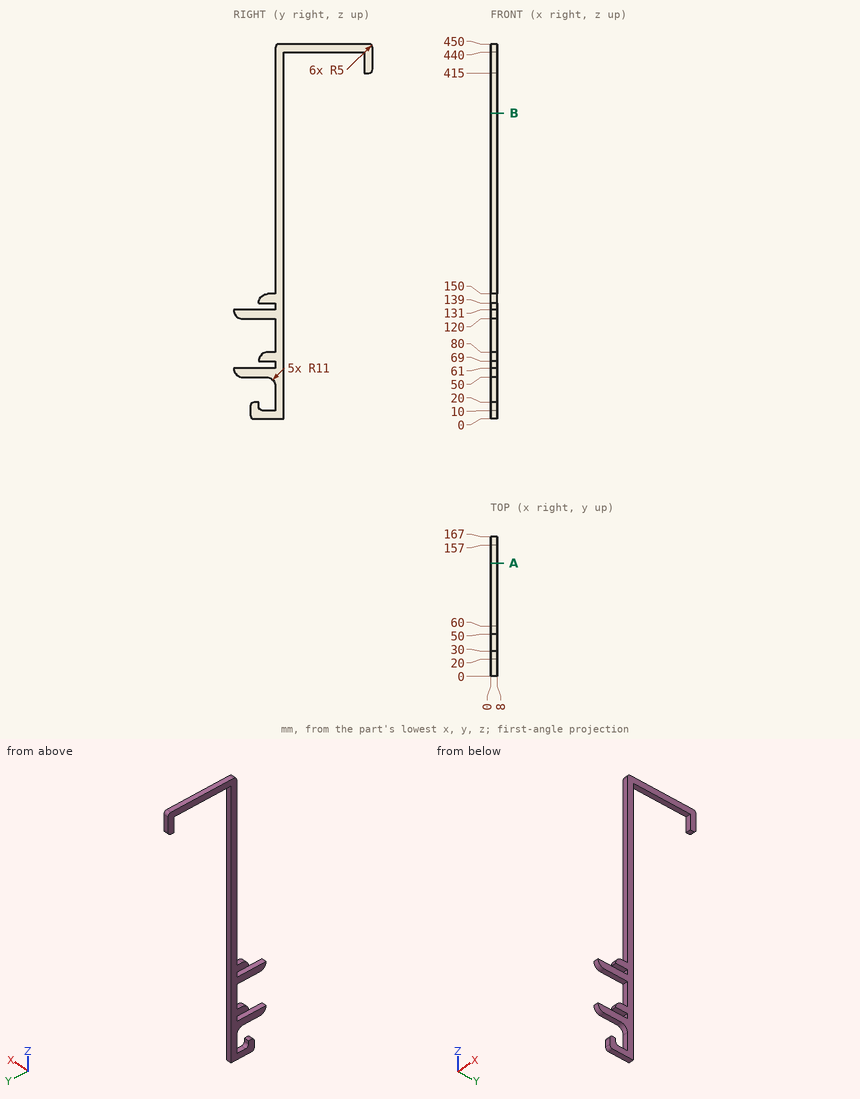
Design review of the part shown in the three views and the two pictorial views. Dimensions are in mm from the part's minimum x, y and z. Coordinates: 2 decimals unless noted, no trailing zeros. Loops run counter-clockwise (first coordinate to the right, second up) from the corner with the lowest first, then second, coordinate; pieces in that order, holes last.
Q1. We need section B-B on z = 367. State the section outline as (x, y) points, and give its area (3 significant figures).
Reported:
outline: (0, 50) - (8, 50) - (8, 60) - (0, 60) - close
area: 80.0 mm2
Q2. For pin 1 (3 mm diameter, centred on x = 5, y = 132.5, fed in from -Z); pin 2 (4 mm diameter, centred on x = 3.5, y = 160.5, fed in from -Z); pin 3 (2.5 mm diameter, centred on x = 4, z = 18, fed in from +Y), all flat-tipped, find the tip position at first contact; note any pin that passes through.
Reported:
pin 1: stops at z = 440
pin 2: stops at z = 415
pin 3: stops at y = 60
Q3. We need section A-A on y = 135.5. State the section outline as (x, z) points.
Reported:
outline: (0, 440) - (8, 440) - (8, 450) - (0, 450) - close
Q4. To check wall thickness, follow line 1 (Z direction, x = 6.25, y = 27); line 2 (Y direction, x = 0.5, z = 427); line 3 (Z direction, x = 6.75, y = 19.5). State the ranges of each line that lie inside material, in increasing order.
Reported:
line 1: z = 0 to 20, 50 to 61, 120 to 131
line 2: y = 50 to 60, 157 to 167
line 3: z = 50 to 61, 120 to 131
